CAD build for the part. Positions are in the model's coordinates, mm. A direction names the side the tool comes from. Round coordinates to 2 decimals unless told otherwise and drop trailing zeros. Order: outer loops, then holes, each group sorted by start corner. A loop starts at its lowest first (then second) coordinate and runs counter-clockwise, first axis right, second up. Notation, with made-up numbers: M -36,24 L -29,24 A25 ccw -29,60 Z; hole C 64,3 d8. An arc over 180 degrees is marked long. Answer as a JSON object with one key per item and string values.
```python
from build123d import *

# Parameters (mm, degrees)
SKETCH2_R            = 45
BOSS_EXTRUDE1_DEPTH  = 42
SKETCH6_R            = 3.825
CUT_EXTRUDE1_DEPTH   = 16
SKETCH10_R           = 4.796352712
BOSS_EXTRUDE2_DEPTH  = 2
SKETCH11_R           = 4
CUT_EXTRUDE2_DEPTH   = 2
LPATTERN1_COUNT      = 3
LPATTERN1_PITCH      = 18
LPATTERN1_COUNT_DIR2 = 3
LPATTERN1_PITCH_DIR2 = 18
LPATTERN2_COUNT      = 3
LPATTERN2_PITCH      = 18
LPATTERN2_COL_COUNT  = 3
LPATTERN2_COL_PITCH  = 18
LPATTERN3_COUNT      = 3
LPATTERN3_PITCH      = 18
LPATTERN3_COL_COUNT  = 3
LPATTERN3_COL_PITCH  = 18
LPATTERN4_COUNT      = 3
LPATTERN4_PITCH      = 18
LPATTERN4_COL_COUNT  = 3
LPATTERN4_COL_PITCH  = 18


with BuildPart() as part:
    # Sketch2 → Boss-Extrude1 (new body)
    with BuildSketch(Plane(origin=(0, 0, 0), x_dir=(1, 0, 0), z_dir=(0, 1, 0))):
        with Locations(Location((0, 0, 0), (0, 0, 90))):
            Circle(SKETCH2_R)
    extrude(amount=BOSS_EXTRUDE1_DEPTH)

    # Sketch6 → Cut-Extrude1 (cut)
    with BuildSketch(Plane(origin=(0, 42, 0), x_dir=(1, 0, 0), z_dir=(0, 1, 0))):
        with Locations(Location((0, 0, 0), (0, 0, 270))):
            Circle(SKETCH6_R)
    cut_extrude1 = extrude(amount=-CUT_EXTRUDE1_DEPTH, mode=Mode.SUBTRACT)

    # Sketch9 → CSK for M5 Countersunk Flat Head Screw1 (revolve, cut)
    with BuildSketch(Plane(origin=(0, 26, 0), x_dir=(0, 0, 1), z_dir=(1, 0, 0))):
        Polygon((0, 0), (0, 15.29228064), (2.65, 13.7), (2.65, 2.55), (5.2, 0), align=None)
    csk_for_m5_countersunk_flat_head_screw1 = revolve(axis=Axis((0, 32.35, 0), (0, -1, 0)), mode=Mode.SUBTRACT)

    # Sketch10 → Boss-Extrude2 (add)
    with BuildSketch(Plane(origin=(0, 42, 0), x_dir=(1, 0, 0), z_dir=(0, 1, 0))):
        with Locations(Location((0, 0, 0), (0, 0, 270))):
            Circle(SKETCH10_R)
    boss_extrude2 = extrude(amount=BOSS_EXTRUDE2_DEPTH)

    # Sketch11 → Cut-Extrude2 (cut)
    with BuildSketch(Plane(origin=(0, 44, 0), x_dir=(1, 0, 0), z_dir=(0, 1, 0))):
        with Locations(Location((0, 0, 0), (0, 0, 270))):
            Circle(SKETCH11_R)
    cut_extrude2 = extrude(amount=-CUT_EXTRUDE2_DEPTH, mode=Mode.SUBTRACT)

    # LPattern1: Cut-Extrude1, CSK for M5 Countersunk Flat Head Screw1, Boss-Extrude2, Cut-Extrude2 3 × 3
    with Locations(*[Vector(1, 0, 0) * (i * LPATTERN1_PITCH) + Vector(-1, 0, 0) * (j * LPATTERN1_PITCH_DIR2) for i in range(LPATTERN1_COUNT) for j in range(LPATTERN1_COUNT_DIR2) if (i, j) != (0, 0)]):
        add(cut_extrude1, mode=Mode.SUBTRACT)
        add(csk_for_m5_countersunk_flat_head_screw1, mode=Mode.SUBTRACT)
        add(boss_extrude2)
        add(cut_extrude2, mode=Mode.SUBTRACT)

    # LPattern2: Cut-Extrude1, CSK for M5 Countersunk Flat Head Screw1, Boss-Extrude2, Cut-Extrude2 ×3
    with Locations(*[(0, 0, -i * LPATTERN2_PITCH) for i in range(1, LPATTERN2_COUNT)]):
        add(cut_extrude1, mode=Mode.SUBTRACT)
        add(csk_for_m5_countersunk_flat_head_screw1, mode=Mode.SUBTRACT)
        add(boss_extrude2)
        add(cut_extrude2, mode=Mode.SUBTRACT)

    # LPattern2 col: Cut-Extrude1, CSK for M5 Countersunk Flat Head Screw1, Boss-Extrude2, Cut-Extrude2 ×3
    with Locations(*[(0, 0, i * LPATTERN2_COL_PITCH) for i in range(1, LPATTERN2_COL_COUNT)]):
        add(cut_extrude1, mode=Mode.SUBTRACT)
        add(csk_for_m5_countersunk_flat_head_screw1, mode=Mode.SUBTRACT)
        add(boss_extrude2)
        add(cut_extrude2, mode=Mode.SUBTRACT)

    # LPattern3: Cut-Extrude1, CSK for M5 Countersunk Flat Head Screw1, Boss-Extrude2, Cut-Extrude2 ×3
    with Locations(*[Vector(-0.7071067811865487, 0, 0.7071067811865464) * (i * LPATTERN3_PITCH) for i in range(1, LPATTERN3_COUNT)]):
        add(cut_extrude1, mode=Mode.SUBTRACT)
        add(csk_for_m5_countersunk_flat_head_screw1, mode=Mode.SUBTRACT)
        add(boss_extrude2)
        add(cut_extrude2, mode=Mode.SUBTRACT)

    # LPattern3 col: Cut-Extrude1, CSK for M5 Countersunk Flat Head Screw1, Boss-Extrude2, Cut-Extrude2 ×3
    with Locations(*[Vector(0.7071067811865487, 0, -0.7071067811865464) * (i * LPATTERN3_COL_PITCH) for i in range(1, LPATTERN3_COL_COUNT)]):
        add(cut_extrude1, mode=Mode.SUBTRACT)
        add(csk_for_m5_countersunk_flat_head_screw1, mode=Mode.SUBTRACT)
        add(boss_extrude2)
        add(cut_extrude2, mode=Mode.SUBTRACT)

    # LPattern4: Cut-Extrude1, CSK for M5 Countersunk Flat Head Screw1, Boss-Extrude2, Cut-Extrude2 ×3
    with Locations(*[Vector(0.7071067811865488, 0, 0.7071067811865462) * (i * LPATTERN4_PITCH) for i in range(1, LPATTERN4_COUNT)]):
        add(cut_extrude1, mode=Mode.SUBTRACT)
        add(csk_for_m5_countersunk_flat_head_screw1, mode=Mode.SUBTRACT)
        add(boss_extrude2)
        add(cut_extrude2, mode=Mode.SUBTRACT)

    # LPattern4 col: Cut-Extrude1, CSK for M5 Countersunk Flat Head Screw1, Boss-Extrude2, Cut-Extrude2 ×3
    with Locations(*[Vector(-0.7071067811865488, 0, -0.7071067811865462) * (i * LPATTERN4_COL_PITCH) for i in range(1, LPATTERN4_COL_COUNT)]):
        add(cut_extrude1, mode=Mode.SUBTRACT)
        add(csk_for_m5_countersunk_flat_head_screw1, mode=Mode.SUBTRACT)
        add(boss_extrude2)
        add(cut_extrude2, mode=Mode.SUBTRACT)


solid = part.part
```
Item 1: Drop flat-ended pins along their axis: pin 1 Ø8.5 at (x, z) = (20, 2) entering from -Y; pin 2 Ø4 at (y, z) = (11, -0.5) entering from -X; pin 3 Ø6 at (x, z) = (18, 0) entering from +Y; pin 4 Ø6 at (y, z) = (8, 32.5) entering from +X. Give the stop position or say it passes through.
Worked answers:
{"pin 1": "stops at y = 0", "pin 2": "stops at x = -45", "pin 3": "stops at y = 23.8", "pin 4": "stops at x = 33.98"}
Item 2: Saw through at A-A on y = 32. State how many separate pieces and enclosed holes the cut face has, and give its area (3 significant figures).
Worked answers:
{"separate pieces": "1", "enclosed holes": "17", "area": "5,580 mm2"}
Item 3: Wall check: line 1 along Z through (x, y) = (22, 27.5); line 2 along X through (y, z) = (23.5, 25); line 3 along X through (y, z) = (14, -13). Give the ranges that are in metal, low to high. Write a range as [from, to].
Worked answers:
{"line 1": "z = [-39.26, -27.1], [-23.82, 23.82], [27.1, 39.26]", "line 2": "x = [-37.42, -28.12], [-22.79, 22.79], [28.12, 37.42]", "line 3": "x = [-43.08, -15.36], [-10.09, 10.09], [15.36, 43.08]"}
Item 4: Saw through at B-B on y = 9. List the corners of the cut face in (x, z).
Worked answers:
{"outline": "C 0,0 d90"}
Item 5: 3-axis set-ups, long thin cutter, end or side, ignore diameter. For faces 1 (the cylindrical face through (-27.69, 17.95, 26.88)), 2 (the flat face through (-3, 44, -21)), 3 (the conical face through (26.53, 23.61, -22.86)): which of +Z, -Z, +X, -X, +Y, -Y reach the whole face in a straight line?
Worked answers:
{"face 1": "+Y", "face 2": "+Z, -Z, +X, -X, +Y", "face 3": "none"}
Item 6: Two-plate mould, pull along Y, no slides. Class faces 4 (the cylindrical face through (-9.49, 42.99, 9.19)), 5 (the flat face through (23, 26, 22)), 6 (the flat face through (-3, 44, -39)): released by +Y, released by -Y, zero draft, split by the parting line, or undercut.
Worked answers:
{"face 4": "zero draft", "face 5": "undercut", "face 6": "released by +Y"}
